```python
from build123d import *

# Parameters (mm, degrees)
SWEEP1_PROFILE_R     = 6.35
CUT_SWEEP1_PROFILE_R = 4.7625


with BuildPart() as part:
    # Sweep1: sweep along a curve in space
    with BuildLine() as sweep1_path:
        Line((0, 0, 0), (0, 0, 304.8))
        ThreePointArc((0, 0, 304.8), (0, 14.878975516, 340.721024484), (0, 50.8, 355.6))
        Line((0, 50.8, 355.6), (0, 76.2, 355.6))
    # Sweep1 profile (on start of the path) → Sweep1 (sweep)
    with BuildSketch(Plane.XY):
        Circle(SWEEP1_PROFILE_R)
    sweep(path=sweep1_path.line)

    # Cut-Sweep1: sweep along a curve in space
    with BuildLine() as cut_sweep1_path:
        Line((0, 0, 0), (0, 0, 304.8))
        ThreePointArc((0, 0, 304.8), (0, 14.878975516, 340.721024484), (0, 50.8, 355.6))
        Line((0, 50.8, 355.6), (0, 76.2, 355.6))
    # Cut-Sweep1 profile (on start of the path) → Cut-Sweep1 (sweep, cut)
    with BuildSketch(Plane.XY):
        Circle(CUT_SWEEP1_PROFILE_R)
    sweep(path=cut_sweep1_path.line, mode=Mode.SUBTRACT)


solid = part.part
```
Geometry check sheet. Reference: the model listing, model coordinates, mm. A direction names the side the tool comes from. Give positions to 0.01 mm unless a question says otherwise; leave off trailing zeros. Write each question's results on one line, items separated by ' | '. Start each with the question number.
(1) Scan lines: line 1 (Z direction, x = 0, y = 56.75); line 2 (X direction, y = 69.25, z = 355.6); line 3 (Y direction, x = 0.5, z = 200). Record each from-to range of solid material in increasing order.
(2) Gauge pin test, flat ends, axial feed: P1, Ø5, axis at x = 5, z = 182, coming from the -Y side; P2, Ø7.5, axis at x = 0, y = 0, coming from the +Z side; P3, Ø1, axis at x = -4, y = 47, coming from the +Z side. Record the tip position at first contact, or that the pin passes through.
(3) Mould release check, pull along Y, two halves, no side actions. Record for faces 3 (the face through (-3.78, -2.9, 154.53)), 4 (the face through (-0.8, 63.7, 349.3)), 5 (the face through (-1.38, -6.2, 154.53)): pulls with the +Y half, pulls with the -Y half, needs draft (parallel to the pull), parting line crosses it, or undercut.
(4) Access from +Z, -Z, +X, -X, +Y, -Y to the whole of each face (thin tool, end or side, straight path). Record for faces 1 (the face through (1, 5, 0)), 2 (the face through (-1.03, 63.68, 360.25)).
Answer below:
1) line 1: 349.25 to 350.84, 360.36 to 361.95 | line 2: -6.35 to -4.76, 4.76 to 6.35 | line 3: -6.33 to -4.74, 4.74 to 6.33
2) P1: y = -5.84 | P2: z = 337.24 | P3: z = 360.77
3) face 3: undercut | face 4: needs draft | face 5: parting line crosses it
4) face 1: -Z, +X, -X, +Y, -Y | face 2: +Y
